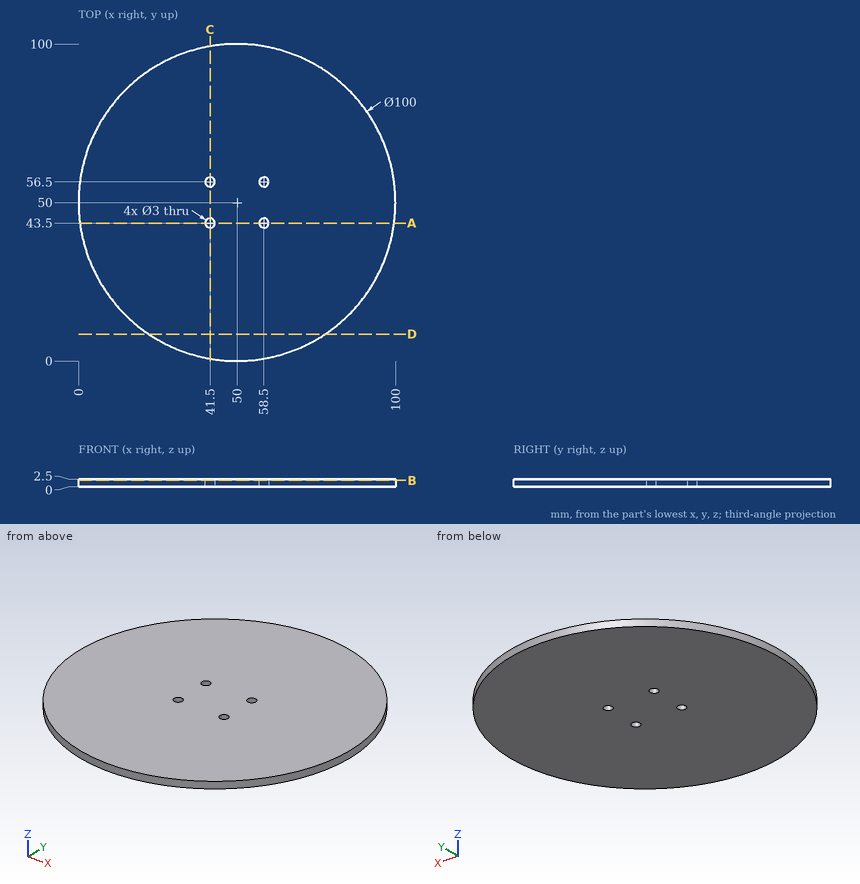
Geometry: see drawing. Coordinates: mm, zero at the bounding-box minimum. Give positions to 0.01 mm unless a question says otherwise; leave off trailing zeros. Order: outer loops, then holes, each group sorted by start corner. A loop starts at its lowest first (then second) coordinate and runs counter-clockwise, first axis right, second up. Notation, with made-up numbers: (71.25, 35) -> (103.25, 35) arc R29 ccw to (103.25, 55) -> close; hole circle Ø9 at (-34.5, 18). An arc over 180 degrees is marked (long way). Write each question's results on one line, items separated by ' | '.
1) Cut plane B-B (z = 2.05). Output: boundary loops of the cut face in (x, y), and give its area (3 significant figures).
Geometry says:
outline: circle Ø100 at (50, 50); hole circle Ø3 at (41.5, 43.5); hole circle Ø3 at (41.5, 56.5); hole circle Ø3 at (58.5, 43.5); hole circle Ø3 at (58.5, 56.5) | area: 7,830 mm²
2) Cut plane D-D (y = 8.5). Output: boundary loops of the cut face in (x, z).
Geometry says:
outline: (22.11, 0) -> (77.89, 0) -> (77.89, 2.5) -> (22.11, 2.5) -> close
3) First-contact query: pin 1 Ø4 at (x, y) = (41.5, 56.5) entering from +Z; pin 2 Ø2.5 at (x, y) = (41.5, 43.5) entering from -Z; pin 3 Ø1 at (x, z) = (52, 1) entering from +Y; pin 4 Ø1.5 at (x, z) = (33, 2) entering from +Y. Flat tips, straight axial feed; report the tip coordinate or a pass-through.
Geometry says:
pin 1: stops at z = 2.5 | pin 2: passes through | pin 3: stops at y = 99.98 | pin 4: stops at y = 97.29
4) Cut plane A-A (y = 43.5). Output: boundary loops of the cut face in (x, z).
Geometry says:
outline: (0.42, 0) -> (40, 0) -> (40, 2.5) -> (0.42, 2.5) -> close; (43, 0) -> (57, 0) -> (57, 2.5) -> (43, 2.5) -> close; (60, 0) -> (99.58, 0) -> (99.58, 2.5) -> (60, 2.5) -> close
5) Cut plane C-C (x = 41.5). Output: boundary loops of the cut face in (y, z), and give its area (3 significant figures).
Geometry says:
outline: (0.73, 0) -> (42, 0) -> (42, 2.5) -> (0.73, 2.5) -> close; (45, 0) -> (55, 0) -> (55, 2.5) -> (45, 2.5) -> close; (58, 0) -> (99.27, 0) -> (99.27, 2.5) -> (58, 2.5) -> close | area: 231 mm²
6) Line query: line 1 along Y through (x, z) = (41.5, 0.6); line 2 along X through (y, z) = (44.5, 1.3); line 3 along Y through (x, z) = (42.5, 0.8). Output: solid intervals per line, ascending.
Geometry says:
line 1: y = 0.73 to 42, 45 to 55, 58 to 99.27 | line 2: x = 0.3 to 40.38, 42.62 to 57.38, 59.62 to 99.7 | line 3: y = 0.57 to 42.38, 44.62 to 55.38, 57.62 to 99.43
